Work out the finished part from the listing and answer in its coordinate system (mm). Give positions to 0.01 mm unless a question says otherwise; leave off trailing zeros. Loops run counter-clockwise (first coordinate to the right, second up) from the corner with the lowest first, then second, coordinate; pieces in that order, holes last. Notation, with made-up numbers: (-25, -27.5) - (23, -27.5) arc R22 cw to (23, -1.5) - close; hole circle Ø5 at (23.25, 76.25). An arc over 180 degrees is marked (long way). One line per item, written item: value.
from build123d import *

# Parameters (mm, degrees)
F0_W     = 15
F0_H     = 15
F1_DEPTH = 105
F3_DEPTH = 105
F5_DEPTH = 105
F7_DEPTH = 105


with BuildPart() as f1:
    # F0 (on Top) → F1 (new body)
    with BuildSketch(Plane.XY):
        with Locations((-3.8708411157, 2.5643814198)):
            Rectangle(F0_W, F0_H)
    extrude(amount=F1_DEPTH)

    # F2 (on face) → F3 (cut)
    with BuildSketch(Plane.XY.offset(105)):
        with BuildLine():
            ThreePointArc((-11.3708411157, 0.8323306122), (-9.3708411157, 0.8323306122), (-8.3708411157, 2.5643814198))
            ThreePointArc((-8.3708411157, 2.5643814198), (-9.3708411157, 4.2964322274), (-11.3708411157, 4.2964322274))
            Line((-11.3708411157, 4.2964322274), (-11.3708411157, 0.8323306122))
        make_face()
    extrude(amount=-F3_DEPTH, mode=Mode.SUBTRACT)

    # F4 (on face) → F5 (cut)
    with BuildSketch(Plane.XY.offset(105)):
        with BuildLine():
            ThreePointArc((-5.6028919233, 10.0643814198), (-4.3884792059, 7.1325297672), (-1.8708411157, 9.0643814198))
            ThreePointArc((-1.8708411157, 9.0643814198), (-1.9389894631, 9.58201951), (-2.1387903081, 10.0643814198))
            Line((-2.1387903081, 10.0643814198), (-5.6028919233, 10.0643814198))
        make_face()
    extrude(amount=-F5_DEPTH, mode=Mode.SUBTRACT)

    # F6 (on face) → F7 (cut)
    with BuildSketch(Plane.XY.offset(105)):
        with BuildLine():
            Line((-5.6028919233, -4.9356185802), (-2.1387903081, -4.9356185802))
            ThreePointArc((-2.1387903081, -4.9356185802), (-1.9389894631, -4.4532566704), (-1.8708411157, -3.9356185802))
            ThreePointArc((-1.8708411157, -3.9356185802), (-4.3884792059, -2.0037669276), (-5.6028919233, -4.9356185802))
        make_face()
        with BuildLine():
            Line((3.6291588843, 0.8323306122), (3.6291588843, 4.2964322274))
            ThreePointArc((3.6291588843, 4.2964322274), (0.6291588843, 2.5643814198), (3.6291588843, 0.8323306122))
        make_face()
    extrude(amount=-F7_DEPTH, mode=Mode.SUBTRACT)


solid = f1.part
1. Section B-B (z = 59) is taken. Write down the section's boundary in (x, y), and give its area (3 significant figures).
Output:
outline: (-11.37, -4.94) - (-5.6, -4.94) arc R2 cw (long way) to (-2.14, -4.94) - (3.63, -4.94) - (3.63, 0.83) arc R2 cw (long way) to (3.63, 4.3) - (3.63, 10.06) - (-2.14, 10.06) arc R2 cw (long way) to (-5.6, 10.06) - (-11.37, 10.06) - (-11.37, 4.3) arc R2 cw (long way) to (-11.37, 0.83) - close
area: 185 mm²
2. Section A-A (x = 2.5) is taken. Write down the section's boundary in (y, z).
Output:
outline: (-4.94, 0) - (0.57, 0) - (0.57, 105) - (-4.94, 105) - close; (4.56, 0) - (10.06, 0) - (10.06, 105) - (4.56, 105) - close
3. Section D-D (x = -3) is taken. Write down the section's boundary in (y, z), and give its area (3 significant figures).
Output:
outline: (-2.14, 0) - (7.26, 0) - (7.26, 105) - (-2.14, 105) - close
area: 987 mm²
4. Section C-C (x = -9.5) is taken. Write down the section's boundary in (y, z).
Output:
outline: (-4.94, 0) - (0.76, 0) - (0.76, 105) - (-4.94, 105) - close; (4.36, 0) - (10.06, 0) - (10.06, 105) - (4.36, 105) - close
5. Find the intervals of material crossed by line 1 along X through (y, z) = (9, 100.5); line 2 along X through (y, z) = (0.75, 10.5); line 3 along X through (y, z) = (8.5, 29), in increasing order.
Output:
line 1: x = -11.37 to -5.87, -1.87 to 3.63
line 2: x = -11.37 to -11.21, -9.53 to 1.79, 3.47 to 3.63
line 3: x = -11.37 to -5.79, -1.95 to 3.63
6. The mould has two halves that part along Z. Classify faces 1 (the flat face through (-4, 3, 105)), 2 (the flat face through (-9, 10.064, 52)), 3 (the flat face through (-4, 3, 0)): released by +Z, released by -Z, zero draft, split by the parting line, or undercut.
Output:
face 1: released by +Z
face 2: zero draft
face 3: released by -Z
7. A flat-ended cylindrical pin translates along its axis: pin 1 Ø3.5 at (x, y) = (2.63, 2.56) entering from +Z. Find the tip coordinate at first contact, or state that the pin passes through.
Output:
pin 1: passes through
